Could you check a few things on this model? Use its own coordinates, in mm. A direction names the side the tool comes from. Round coordinates to 2 decimals unless told otherwise and drop trailing zeros. Loops run counter-clockwise (first coordinate to the right, second up) from the corner with the lowest first, then second, coordinate; pieces in that order, holes last. Notation, with made-up numbers: M 34,39 L 40,39 A19 ccw 40,67 Z; hole C 46.5,5.5 d1. An arc over 180 degrees is marked long. Answer in a Markdown table with one row per item.
```python
from build123d import *

# Parameters (mm, degrees)
F1_DEPTH  = 31.75
F3_DEPTH  = 31.75
F7_DEPTH  = 19.05
F9_W      = 50.8
F9_H      = 19.05
F10_DEPTH = 31.75
F11_DEPTH = 19.05
F13_DEPTH = 19.05
F14_DEPTH = 12.7
F15_DEPTH = 12.7
F17_DEPTH = 12.7
F18_R     = 6.35
F19_DEPTH = 31.75
F20_R     = 3.175
F21_DEPTH = 6.35
F23_DEPTH = 6.35
F25_DEPTH = 6.35


with BuildPart() as f1:
    # F0 (on Front) → F1 (new body)
    with BuildSketch(Plane.XZ):
        Polygon((0, 6.35), (0, 0), (50.8, 0), (50.8, 6.35), (38.1, 6.35), (38.1, 57.15), (12.7, 57.15), (12.7, 6.35), align=None)
    extrude(amount=F1_DEPTH)

    # F2 (on face) → F3 (cut)
    with BuildSketch(Plane.XZ.offset(31.75)):
        with BuildLine():
            ThreePointArc((12.7, 44.45), (16.4197438789, 53.4302561211), (25.4, 57.15))
            Line((25.4, 57.15), (12.7, 57.15))
            Line((12.7, 57.15), (12.7, 44.45))
        make_face()
        with BuildLine():
            ThreePointArc((25.4, 57.15), (34.3802561211, 53.4302561211), (38.1, 44.45))
            Line((38.1, 44.45), (38.1, 57.15))
            Line((38.1, 57.15), (25.4, 57.15))
        make_face()
    extrude(amount=-F3_DEPTH, mode=Mode.SUBTRACT)

    # F5 (on face) → F7 (cut)
    with BuildSketch(Plane.XZ.offset(31.75)):
        with BuildLine():
            ThreePointArc((38.1, 44.45), (34.3802561211, 35.4697438789), (25.4, 31.75))
            Line((25.4, 31.75), (38.1, 31.75))
            Line((38.1, 31.75), (38.1, 44.45))
        make_face()
    extrude(amount=-F7_DEPTH, mode=Mode.SUBTRACT)

    # F9 (on face) → F10 (cut)
    with BuildSketch(Plane(origin=(0, 0, 0), x_dir=(1, 0, 0), z_dir=(0, 0, -1))):
        with Locations((25.4, 22.225)):
            Rectangle(F9_W, F9_H)
    extrude(amount=-F10_DEPTH, mode=Mode.SUBTRACT)

    # F8 (on face) → F11 (cut)
    with BuildSketch(Plane.XZ.offset(31.75)):
        with BuildLine():
            Line((12.7, 31.75), (25.4, 31.75))
            ThreePointArc((25.4, 31.75), (16.4197438789, 35.4697438789), (12.7, 44.45))
            Line((12.7, 44.45), (12.7, 31.75))
        make_face()
    extrude(amount=-F11_DEPTH, mode=Mode.SUBTRACT)

    # F12 (on face) → F13 (join)
    with BuildSketch(Plane.XZ.offset(12.7)):
        Polygon((38.1, 6.35), (12.7, 6.35), (0, 6.35), (0, 0), (50.8, 0), (50.8, 6.35), align=None)
    extrude(amount=F13_DEPTH)

    # F14 (add): a face of the model
    f14_faces = [f1.faces().sort_by_distance(p)[0] for p in [
        (12.7, -6.35, 25.4),
    ]]
    extrude(f14_faces, amount=F14_DEPTH)

    # F15 (add): a face of the model
    f15_faces = [f1.faces().sort_by_distance(p)[0] for p in [
        (38.1, -6.35, 25.4),
    ]]
    extrude(f15_faces, amount=F15_DEPTH)

    # F16 (on face) → F17 (cut)
    with BuildSketch(Plane.XZ.offset(12.7)):
        with BuildLine():
            Line((0, 44.45), (0, 6.35))
            ThreePointArc((0, 6.35), (9.4413894262, 24.3695368579), (12.7, 44.45))
            Line((12.7, 44.45), (0, 44.45))
        make_face()
        with BuildLine():
            ThreePointArc((38.1, 44.45), (41.3586105738, 24.3695368579), (50.8, 6.35))
            Line((50.8, 6.35), (50.8, 44.45))
            Line((50.8, 44.45), (38.1, 44.45))
        make_face()
    extrude(amount=-F17_DEPTH, mode=Mode.SUBTRACT)

    # F18 (on face) → F19 (cut)
    with BuildSketch(Plane.XZ.offset(31.75)):
        with Locations((25.4, 44.4756895304)):
            Circle(F18_R)
    extrude(amount=-F19_DEPTH, mode=Mode.SUBTRACT)

    # F20 (on face) → F21 (cut)
    with BuildSketch(Plane.XY.offset(6.35)):
        with Locations((44.45, -25.4)):
            Circle(F20_R)
        with Locations((6.35, -25.4)):
            Circle(F20_R)
    extrude(amount=-F21_DEPTH, mode=Mode.SUBTRACT)

    # F22 (on face) → F23 (cut)
    with BuildSketch(Plane.XY.offset(6.35)):
        with BuildLine():
            ThreePointArc((6.35, -31.75), (1.8598719395, -29.8901280605), (0, -25.4))
            Line((0, -25.4), (0, -31.75))
            Line((0, -31.75), (6.35, -31.75))
        make_face()
    extrude(amount=-F23_DEPTH, mode=Mode.SUBTRACT)

    # F24 (on face) → F25 (cut)
    with BuildSketch(Plane.XY.offset(6.35)):
        with BuildLine():
            ThreePointArc((50.8, -25.4), (48.9401280605, -29.8901280605), (44.45, -31.75))
            Line((44.45, -31.75), (50.8, -31.75))
            Line((50.8, -31.75), (50.8, -25.4))
        make_face()
    extrude(amount=-F25_DEPTH, mode=Mode.SUBTRACT)


solid = f1.part
```
1) Which directions (+Z, -Z, +X, -X, +Y, -Y) give clear straight access to the entire face, cutting with the end or side of a thin tool? Please do faces 4 (the face through (26, -22, 6.35)), 5 (the face through (9.35, -6.44, 24.1)).
Computed:
| item | result |
|---|---|
| face 4 | +X, -X, -Y |
| face 5 | +Z, -X, +Y, -Y |
2) I want a section at D-D, the plane z = 33. Please give me the cut outline in (x, y).
Computed:
| item | result |
|---|---|
| outline | M 11.66,-12.7 L 19.91,-12.7 L 19.91,-31.75 L 30.89,-31.75 L 30.89,-12.7 L 39.14,-12.7 L 39.14,0 L 11.66,0 Z |
3) I want a section at B-B, the plane y = -7. Please give me the cut outline in (x, z), plus the area to 3 significant figures.
Computed:
| item | result |
|---|---|
| outline | M 0,0 L 50.8,0 L 50.8,6.35 A63.5 cw 38.1,44.45 A12.7 ccw 12.7,44.45 A63.5 cw 0,6.35 Z; hole C 25.4,44.48 d12.7 |
| area | 1,730 mm² |
4) I want a section at C-C, the plane x = 27. Please give me the cut outline in (y, z), plus the area to 3 significant figures.
Computed:
| item | result |
|---|---|
| outline | M -31.75,0 L 0,0 L 0,38.33 L -31.75,38.33 L -31.75,31.85 L -12.7,31.85 L -12.7,6.35 L -31.75,6.35 Z; M -31.75,50.62 L 0,50.62 L 0,57.05 L -31.75,57.05 Z |
| area | 935 mm² |
5) I need wall thicknesses on line 1 (X direction, y = -25, z = 2); line 2 (Z direction, x = 22, y = -30); line 3 (Z direction, x = 25, y = -6.5). Which ranges of each line are inside material? Lowest first, please.
Computed:
| item | result |
|---|---|
| line 1 | x = 0 to 3.2, 9.5 to 41.3, 47.6 to 50.8 |
| line 2 | z = 0 to 6.35, 32.21 to 39.11, 49.84 to 56.69 |
| line 3 | z = 0 to 38.14, 50.81 to 57.14 |
6) Will these pins go through, and if not, where does the flat tip stop? P1, Ø5.5, axis at x = 16.5, y = -25.5, coming from the +Z side; P2, Ø6, axis at x = 11.5, z = 32.5, coming from the -Y side; P3, Ø2, axis at y = -7, z = 38.5, coming from the +X side.
Computed:
| item | result |
|---|---|
| P1 | stops at z = 55.56 |
| P2 | stops at y = -12.7 |
| P3 | stops at x = 38.48 |
7) If we mould it in two halves opening along Y, with no side actions, what happens to faces 1 (the face through (1.91, -29.94, 3.22)), 2 (the face through (25, 0, 22)), 3 (the face through (42.11, -23.254, 3.219))? For each: released by +Y, released by -Y, zero draft, split by the parting line, or undercut.
Computed:
| item | result |
|---|---|
| face 1 | released by -Y |
| face 2 | released by +Y |
| face 3 | undercut |
8) I want a section at A-A, the plane y = -24. Please give me the cut outline in (x, z), plus the area to 3 significant figures.
Computed:
| item | result |
|---|---|
| outline | M 0,0 L 3.5,0 L 3.5,6.35 L 0,6.35 Z; M 9.2,0 L 41.6,0 L 41.6,6.35 L 9.2,6.35 Z; C 25.4,44.45 d25.4; M 47.3,0 L 50.8,0 L 50.8,6.35 L 47.3,6.35 Z; hole C 25.4,44.48 d12.7 |
| area | 630 mm² |
